The model under review builds one solid part; all positions refer to its coordinate system, in mm. A direction names the side the tool comes from. Coordinates: 2 decimals unless noted, no trailing zeros. Order: outer loops, then holes, each group sorted by start corner. A loop starts at its lowest first (then second) coordinate and runs counter-clockwise, first axis right, second up. Notation, with made-up numbers: (66.25, 2.5) -> (78.25, 2.5) arc R15 cw to (78.25, 24.5) -> close; hole circle Ø9 at (-38, 61.25). An arc over 180 degrees is marked (long way). Answer as CSV lines item,"result". Start each with the question number.
from build123d import *

# Parameters (mm, degrees)
F1_DEPTH = 25


with BuildPart() as f1:
    # F0 (on Front) → F1 (new body, symmetric)
    with BuildSketch(Plane.XZ):
        with BuildLine():
            Line((50, 0), (0, 0))
            Line((0, 0), (0, 30))
            ThreePointArc((0, 30), (-21.213203, 21.213203), (-30, 0))
            Line((-30, 0), (-30, -20))
            ThreePointArc((-30, -20), (10, -30), (50, -20))
            Line((50, -20), (50, 0))
        make_face()
    extrude(amount=F1_DEPTH, both=True)


solid = f1.part
1) Tool access review of faces 1 (the face through (9.42, -0.35, -30)), 2 (the face through (25, 0, 0)): name each direction out of +Z, -Z, +X, -X, +Y, -Y from which nothing blocks a thin tool from reaching the whole face with its end or side.
2) Consider section C-C (z = 10.5). Give the boundary of the cut face in (x, y).
3) Consider section A-A (y = 14). Give the boundary of the cut face in (x, z), plus the area to 3 significant figures.
4) Wall thickness on L1, parallel to Z at x = -12, y = -4; L2, parallel to X at y = -21.5, z = 0.5; L3, parallel to X at y = 5, z = 15: over which ranges is each line inside the solid? List them lowest first. Write a range as [from, to].
5) Insertion check: pin 1 Ø5 at (x, y) = (7.5, -12) entering from -Z; pin 2 Ø10 at (x, y) = (41, -12) entering from +Z; pin 3 Ø4 at (x, y) = (-4, 4) entering from +Z. Each pin has a flat end and moves straight along its axis. Give the tip position at first contact, or say it passes through.
6) Consider section B-B (x = -18.5). Give the boundary of the cut face in (y, z), plus the area to 3 significant figures.
Result:
1,face 1,"-Z, +Y, -Y"
1,face 2,"+Z, +X, +Y, -Y"
2,outline,"(-28.1, -25) -> (0, -25) -> (0, 25) -> (-28.1, 25) -> close"
3,outline,"(-30, -20) arc R85 ccw to (50, -20) -> (50, 0) -> (0, 0) -> (0, 30) arc R30 ccw to (-30, 0) -> close"
3,area,"2,850 mm2"
4,L1,"[-27.1, 27.5]"
4,L2,"[-30, 0]"
4,L3,"[-25.98, 0]"
5,pin 1,"z = -30"
5,pin 2,"z = 0"
5,pin 3,"z = 29.93"
6,outline,"(-25, -25.08) -> (25, -25.08) -> (25, 23.62) -> (-25, 23.62) -> close"
6,area,"2,430 mm2"
